Geometry check sheet. Reference: the model listing, model coordinates, mm. A direction names the side the tool comes from. Round coordinates to 2 decimals unless told otherwise and drop trailing zeros. Loops run counter-clockwise (first coordinate to the right, second up) from the corner with the lowest first, then second, coordinate; pieces in that order, holes last. Notation, with made-up numbers: M 77.5,-8.5 L 134.5,-8.5 A21 cw 134.5,-2.5 Z; hole C 69.5,-20.5 d11. An arc over 180 degrees is marked long. Use one line per item in the form item = value. Start each with the question number.
1. Cross-section at A-A (z = -7.25). Record the boundary of the cut face in (x, y).
2. Cross-section at C-C (z = 0). State how many separate pieces and enclosed holes the cut face has, then the cut area to 3 significant figures.
3. Draft check along X on faces 1 (the flat face through (13, 2, -4)), 2 (the flat face through (-14, 2, -0.8)), 3 (the flat face through (4, 2, -13)). Enter one of: pulls with the +X half, pulls with the -X half, needs draft (parallel to the pull), parting line crosses it, or undercut.
4. Go/stop test with flat-tipped pins: pin 1 (4.5 mm diameter, centred on x = 0, z = 0, fed in from +Y); pin 2 (1.6 mm diameter, centred on x = -14.5, y = 2.5, fed in from -Z); pin 3 (1.2 mm diameter, centred on x = -17.5, y = 1.5, fed in from -Z); pin 4 (0.7 mm diameter, centred on y = 3, z = 2, fed in from -X). Record where each tip stops, or that it passes through.
5. Set-up check for faces 4 (the flat face through (0, 2, 4)), 5 (the cylindrical face through (-13.6, 2, 0)), 6 (the cylindrical face through (0.1, 3.6, -19)): record each of +Z, -Z, +X, -X, +Y, -Y from which the full face is reachable in a straight line by a thin tool's end or side.
6. Cross-section at B-B (x = 7). Record the boundary of the cut face in (y, z), then the cut area to 3 significant figures.
7. Material ranges on line 1 (X direction, y = 3.5, z = 0); line 2 (Z direction, x = 16, y = 0.65); line 3 (X direction, y = 1.75, z = 0), recorded low to high.
```python
from build123d import *

# Parameters (mm, degrees)
SKETCH_1_R          = 2.4
EXTRUDE_1_DEPTH     = 4
SKETCH_2_R          = 3
CUT_EXTRUDE_1_DEPTH = 0.9
EXTRUDE_START       = -4
EXTRUDE_2_DEPTH     = 4


with BuildPart() as part:
    # 草图1 → 凸台-拉伸1 (new body)
    with BuildSketch(Plane(origin=(0, 0, 0), x_dir=(1, 0, 0), z_dir=(0, 1, 0))):
        with BuildLine():
            Line((-16, 4), (-10.388851415, 4))
            Line((-10.388851415, 4), (-4, 10))
            Line((-4, 10), (-4, 16))
            ThreePointArc((-4, 16), (0, 20), (4, 16))
            Line((4, 16), (4, 10))
            Line((4, 10), (10.388851415, 4))
            Line((10.388851415, 4), (16, 4))
            ThreePointArc((16, 4), (20, 0), (16, -4))
            Line((16, -4), (-16, -4))
            ThreePointArc((-16, -4), (-20, 0), (-16, 4))
        make_face()
        with Locations(Location((16, 0, 0), (0, 0, 270))):
            Circle(SKETCH_1_R, mode=Mode.SUBTRACT)
        with Locations(Location((8, 0, 0), (0, 0, 270))):
            Circle(SKETCH_1_R, mode=Mode.SUBTRACT)
        with Locations(Location((0, 0, 0), (0, 0, 270))):
            Circle(SKETCH_1_R, mode=Mode.SUBTRACT)
        with Locations(Location((-8, 0, 0), (0, 0, 270))):
            Circle(SKETCH_1_R, mode=Mode.SUBTRACT)
        with Locations(Location((-16, 0, 0), (0, 0, 270))):
            Circle(SKETCH_1_R, mode=Mode.SUBTRACT)
        with Locations(Location((0, 8, 0), (0, 0, 270))):
            Circle(SKETCH_1_R, mode=Mode.SUBTRACT)
        with Locations(Location((0, 16, 0), (0, 0, 270))):
            Circle(SKETCH_1_R, mode=Mode.SUBTRACT)
    extrude(amount=EXTRUDE_1_DEPTH)

    # 草图2 → 切除-拉伸1 (cut)
    with BuildSketch(Plane(origin=(0, 4, 0), x_dir=(1, 0, 0), z_dir=(0, 1, 0))):
        with Locations(Location((-8, 0, 0), (0, 0, 270))):
            Circle(SKETCH_2_R)
        with Locations(Location((0, 0, 0), (0, 0, 270))):
            Circle(SKETCH_2_R)
        with Locations(Location((8, 0, 0), (0, 0, 270))):
            Circle(SKETCH_2_R)
        with Locations(Location((0, 8, 0), (0, 0, 270))):
            Circle(SKETCH_2_R)
        with Locations(Location((0, 16, 0), (0, 0, 270))):
            Circle(SKETCH_2_R)
    cut_extrude_1 = extrude(amount=-CUT_EXTRUDE_1_DEPTH, mode=Mode.SUBTRACT)

    # 镜向1: 切除-拉伸1 across plane
    add(cut_extrude_1.mirror(Plane.ZX.offset(2)), mode=Mode.SUBTRACT)

    # 草图4 → 凸台-拉伸2 (add)
    with BuildSketch(Plane(origin=(0, 4, 0), x_dir=(1, 0, 0), z_dir=(0, 1, 0)).offset(EXTRUDE_START)):
        with BuildLine():
            Line((-16.8, 0.8), (-16.8, 2.2627417))
            ThreePointArc((-16.8, 2.2627417), (-17.697056275, 1.697056275), (-18.2627417, 0.8))
            Line((-18.2627417, 0.8), (-16.8, 0.8))
        make_face()
        with BuildLine():
            ThreePointArc((-13.7372583, 0.8), (-14.302943725, 1.697056275), (-15.2, 2.2627417))
            Line((-15.2, 2.2627417), (-15.2, 0.8))
            Line((-15.2, 0.8), (-13.7372583, 0.8))
        make_face()
        with BuildLine():
            Line((-13.7372583, -0.8), (-15.2, -0.8))
            Line((-15.2, -0.8), (-15.2, -2.2627417))
            ThreePointArc((-15.2, -2.2627417), (-14.302943725, -1.697056275), (-13.7372583, -0.8))
        make_face()
        with BuildLine():
            Line((-16.8, -2.2627417), (-16.8, -0.8))
            Line((-16.8, -0.8), (-18.2627417, -0.8))
            ThreePointArc((-18.2627417, -0.8), (-17.697056275, -1.697056275), (-16.8, -2.2627417))
        make_face()
        with BuildLine():
            Line((13.7372583, 0.8), (15.2, 0.8))
            Line((15.2, 0.8), (15.2, 2.2627417))
            ThreePointArc((15.2, 2.2627417), (14.302943725, 1.697056275), (13.7372583, 0.8))
        make_face()
        with BuildLine():
            Line((16.8, 0.8), (18.2627417, 0.8))
            ThreePointArc((18.2627417, 0.8), (17.697056275, 1.697056275), (16.8, 2.2627417))
            Line((16.8, 2.2627417), (16.8, 0.8))
        make_face()
        with BuildLine():
            Line((18.2627417, -0.8), (16.8, -0.8))
            Line((16.8, -0.8), (16.8, -2.2627417))
            ThreePointArc((16.8, -2.2627417), (17.697056275, -1.697056275), (18.2627417, -0.8))
        make_face()
        with BuildLine():
            Line((15.2, -2.2627417), (15.2, -0.8))
            Line((15.2, -0.8), (13.7372583, -0.8))
            ThreePointArc((13.7372583, -0.8), (14.302943725, -1.697056275), (15.2, -2.2627417))
        make_face()
    extrude(amount=EXTRUDE_2_DEPTH)


solid = part.part
```
Reported:
q1.outline = M -6.93,0 L -2.9,0 L -2.9,0.9 L -2.28,0.9 L -2.28,3.1 L -2.9,3.1 L -2.9,4 L -6.93,4 Z; M 2.28,0.9 L 2.9,0.9 L 2.9,0 L 6.93,0 L 6.93,4 L 2.9,4 L 2.9,3.1 L 2.28,3.1 Z
q2.separate_pieces = 6
q2.enclosed_holes = 0
q2.area = 57.5 mm²
q3.face_1 = needs draft
q3.face_2 = undercut
q3.face_3 = pulls with the +X half
q4.pin_1 = through
q4.pin_2 = -4
q4.pin_3 = -3.9
q4.pin_4 = -19.64
q5.face_4 = +Z, +X, -X, +Y, -Y
q5.face_5 = +Y, -Y
q5.face_6 = +Y
q6.outline = M 0,-7.18 L 4,-7.18 L 4,-2.83 L 3.1,-2.83 L 3.1,-2.18 L 0.9,-2.18 L 0.9,-2.83 L 0,-2.83 Z; M 0,2.83 L 0.9,2.83 L 0.9,2.18 L 3.1,2.18 L 3.1,2.83 L 4,2.83 L 4,4 L 0,4 Z
q6.area = 24.9 mm²
q7.line_1 = -20 to -18.4, -13.6 to -11, -5 to -3, 3 to 5, 11 to 13.6, 18.4 to 20
q7.line_2 = -4 to -2.4, 2.4 to 4
q7.line_3 = -20 to -18.4, -13.6 to -10.4, -5.6 to -2.4, 2.4 to 5.6, 10.4 to 13.6, 18.4 to 20
